Autodesk Inventor part; units mm, degrees
ref_plane "YZ Plane" through (0, 0, 0) normal (1, 0, 0) x (0, 1, 0)
ref_plane "XZ Plane" through (0, 0, 0) normal (0, 1, 0) x (-1, 0, 0)
ref_plane "XY Plane" through (0, 0, 0) normal (0, 0, 1) x (1, 0, 0)
sketch "Эскиз1" plane through (0, 0, 0) normal (1, 0, 0) x (0, 1, 0)
  circle A0 centre (0, 0) radius 60
  point P0 (0, -60)
extrude "Выдавливание1" add sketch "Эскиз1" along normal blind 4
sketch "Эскиз2" plane through (4, 0, 0) normal (1, 0, 0) x (0, 0, -1)
  point P0 (0, 0)
  point P1 (0, -60)
sketch "Эскиз3" plane through (4, 0, 0) normal (1, 0, 0) x (0, 0, -1)
  line L0 (0, -92.75) -> (0, 85.4583) construction
  circle A0 centre (0, 0) radius 60 construction
  line L1 (40.5908, -40.3227) -> (46.095, -31.9738)
  line L2 (46.095, -31.9738) -> (42.7554, -29.7722)
  line L3 (42.7554, -29.7722) -> (37.2513, -38.1211)
  line L4 (37.2513, -38.1211) -> (40.5908, -40.3227)
  line L5 (40.5908, -40.3227) -> (42.7554, -29.7722) construction
  line L6 (46.095, -31.9738) -> (37.2513, -38.1211) construction
  line L7 (41.6731, -35.0475) -> (44.4252, -30.873) construction
  line L8 (31.7471, -46.47) -> (48.2596, -21.4233) construction
  line L9 (48.2596, -21.4233) -> (51.5992, -23.6249) construction
  line L10 (51.5992, -23.6249) -> (35.0866, -48.6716) construction
  line L11 (35.0866, -48.6716) -> (31.7471, -46.47) construction
  line L12 (31.7471, -46.47) -> (51.5992, -23.6249) construction
  line L13 (48.2596, -21.4233) -> (35.0866, -48.6716) construction
  circle A1 centre (0, 0) radius 60
  line L14 (48.3995, -11.3168) -> (48.3995, -1.3168)
  line L15 (48.3995, -1.3168) -> (52.3995, -1.3168)
  line L16 (52.3995, -1.3168) -> (52.3995, -11.3168) construction
  line L17 (52.3995, -11.3168) -> (48.3995, -11.3168)
  line L18 (48.3995, -11.3168) -> (52.3995, -1.3168) construction
  line L19 (48.3995, -1.3168) -> (52.3995, -11.3168) construction
  line L20 (48.3995, -21.3168) -> (48.3995, 8.6832) construction
  line L21 (48.3995, 8.6832) -> (52.3995, 8.6832) construction
  line L22 (52.3995, 8.6832) -> (52.3995, -21.3168)
  line L23 (52.3995, -21.3168) -> (48.3995, -21.3168) construction
  line L24 (48.3995, -21.3168) -> (52.3995, 8.6832) construction
  line L25 (48.3995, 8.6832) -> (52.3995, -21.3168) construction
  line L26 (50.3995, -6.3168) -> (50.3995, 8.6832) construction
  line L27 (36.4646, 25.3316) -> (42.4094, 17.2905)
  line L28 (42.4094, 17.2905) -> (45.6259, 19.6684)
  line L29 (45.6259, 19.6684) -> (39.6811, 27.7095)
  line L30 (39.6811, 27.7095) -> (36.4646, 25.3316)
  line L31 (36.4646, 25.3316) -> (45.6259, 19.6684) construction
  line L32 (42.4094, 17.2905) -> (39.6811, 27.7095) construction
  line L33 (30.5198, 33.3727) -> (48.3542, 9.2494) construction
  line L34 (48.3542, 9.2494) -> (51.5707, 11.6273) construction
  line L35 (51.5707, 11.6273) -> (33.7363, 35.7506) construction
  line L36 (33.7363, 35.7506) -> (30.5198, 33.3727) construction
  line L37 (30.5198, 33.3727) -> (51.5707, 11.6273) construction
  line L38 (48.3542, 9.2494) -> (33.7363, 35.7506) construction
  line L39 (41.0453, 22.5) -> (32.1281, 34.5617) construction
  line L40 (10.536, 42.571) -> (20.3099, 40.4564)
  line L41 (20.3099, 40.4564) -> (19.464, 36.5468)
  line L42 (19.464, 36.5468) -> (9.6901, 38.6615)
  line L43 (9.6901, 38.6615) -> (10.536, 42.571)
  line L44 (10.536, 42.571) -> (19.464, 36.5468) construction
  line L45 (20.3099, 40.4564) -> (9.6901, 38.6615) construction
  line L46 (-0.0837, 40.7762) -> (29.2378, 34.4321) construction
  line L47 (29.2378, 34.4321) -> (30.0837, 38.3417) construction
  line L48 (30.0837, 38.3417) -> (0.7622, 44.6857) construction
  line L49 (0.7622, 44.6857) -> (-0.0837, 40.7762) construction
  line L50 (-0.0837, 40.7762) -> (30.0837, 38.3417) construction
  line L51 (29.2378, 34.4321) -> (0.7622, 44.6857) construction
  line L52 (0.3392, 42.7309) -> (15, 39.5589) construction
  line L53 (-20.2765, 33.1516) -> (-11.9215, 38.6465)
  line L54 (-11.9215, 38.6465) -> (-9.7235, 35.3046)
  line L55 (-9.7235, 35.3046) -> (-18.0785, 29.8096)
  line L56 (-18.0785, 29.8096) -> (-20.2765, 33.1516)
  line L57 (-20.2765, 33.1516) -> (-9.7235, 35.3046) construction
  line L58 (-11.9215, 38.6465) -> (-18.0785, 29.8096) construction
  line L59 (-26.4334, 24.3146) -> (-1.3686, 40.7995) construction
  line L60 (-1.3686, 40.7995) -> (-3.5666, 44.1415) construction
  line L61 (-3.5666, 44.1415) -> (-28.6314, 27.6566) construction
  line L62 (-28.6314, 27.6566) -> (-26.4334, 24.3146) construction
  line L63 (-26.4334, 24.3146) -> (-3.5666, 44.1415) construction
  line L64 (-1.3686, 40.7995) -> (-28.6314, 27.6566) construction
  line L65 (-15, 34.2281) -> (-2.4676, 42.4705) construction
  line L66 (-32.897, 9.0632) -> (-30.5956, 18.7948)
  line L67 (-30.5956, 18.7948) -> (-26.703, 17.8742)
  line L68 (-26.703, 17.8742) -> (-29.0044, 8.1427)
  line L69 (-29.0044, 8.1427) -> (-32.897, 9.0632)
  line L70 (-32.897, 9.0632) -> (-26.703, 17.8742) construction
  line L71 (-30.5956, 18.7948) -> (-29.0044, 8.1427) construction
  line L72 (-34.0478, 4.1975) -> (-29.4449, 23.6606) construction
  line L73 (-29.4449, 23.6606) -> (-25.5522, 22.74) construction
  line L74 (-25.5522, 22.74) -> (-30.1551, 3.2769) construction
  line L75 (-30.1551, 3.2769) -> (-34.0478, 4.1975) construction
  line L76 (-34.0478, 4.1975) -> (-25.5522, 22.74) construction
  line L77 (-29.4449, 23.6606) -> (-30.1551, 3.2769) construction
  line L78 (-29.8, 13.4687) -> (-27.4986, 23.2003) construction
  line L79 (-30.1437, 1.6896) -> (-20.3668, -15.7578) construction
  line L80 (-20.3668, -15.7578) -> (-23.8563, -17.7132) construction
  line L81 (-23.8563, -17.7132) -> (-33.6332, -0.2658) construction
  line L82 (-33.6332, -0.2658) -> (-30.1437, 1.6896) construction
  line L83 (-30.1437, 1.6896) -> (-23.8563, -17.7132) construction
  line L84 (-20.3668, -15.7578) -> (-33.6332, -0.2658) construction
  line L85 (-27.6995, -2.6723) -> (-22.811, -11.396)
  line L86 (-22.811, -11.396) -> (-26.3005, -13.3514)
  line L87 (-26.3005, -13.3514) -> (-31.189, -4.6277)
  line L88 (-31.189, -4.6277) -> (-27.6995, -2.6723)
  line L89 (-27.6995, -2.6723) -> (-26.3005, -13.3514) construction
  line L90 (-22.811, -11.396) -> (-31.189, -4.6277) construction
  line L91 (-27, -8.0118) -> (-31.8884, 0.7119) construction
  line L92 (-19.4768, -16.8116) -> (0.1967, -20.411) construction
  line L93 (0.1967, -20.411) -> (-0.5232, -24.3456) construction
  line L94 (-0.5232, -24.3456) -> (-20.1967, -20.7463) construction
  line L95 (-20.1967, -20.7463) -> (-19.4768, -16.8116) construction
  line L96 (-19.4768, -16.8116) -> (-0.5232, -24.3456) construction
  line L97 (0.1967, -20.411) -> (-20.1967, -20.7463) construction
  line L98 (-14.5584, -17.7114) -> (-4.7217, -19.5111)
  line L99 (-4.7217, -19.5111) -> (-5.4416, -23.4458)
  line L100 (-5.4416, -23.4458) -> (-15.2783, -21.6461)
  line L101 (-15.2783, -21.6461) -> (-14.5584, -17.7114)
  line L102 (-14.5584, -17.7114) -> (-5.4416, -23.4458) construction
  line L103 (-4.7217, -19.5111) -> (-15.2783, -21.6461) construction
  line L104 (-10, -20.5786) -> (-19.8367, -18.7789) construction
  line L105 (11.0144, -9.2398) -> (0.2107, -19.6457) construction
  line L106 (0.2107, -19.6457) -> (2.9856, -22.5267) construction
  line L107 (2.9856, -22.5267) -> (13.7893, -12.1208) construction
  line L108 (13.7893, -12.1208) -> (11.0144, -9.2398) construction
  line L109 (11.0144, -9.2398) -> (2.9856, -22.5267) construction
  line L110 (0.2107, -19.6457) -> (13.7893, -12.1208) construction
  line L111 (9.2138, -10.9742) -> (2.0113, -17.9114)
  line L112 (2.0113, -17.9114) -> (4.7862, -20.7923)
  line L113 (4.7862, -20.7923) -> (11.9887, -13.8551)
  line L114 (11.9887, -13.8551) -> (9.2138, -10.9742)
  line L115 (9.2138, -10.9742) -> (4.7862, -20.7923) construction
  line L116 (2.0113, -17.9114) -> (11.9887, -13.8551) construction
  line L117 (7, -15.8832) -> (10.6012, -12.4146) construction
  line L118 (10.3281, -8.9147) -> (8.5366, 0.9236)
  line L119 (8.5366, 0.9236) -> (12.4719, 1.6401)
  line L120 (12.4719, 1.6401) -> (14.2634, -8.1981)
  line L121 (14.2634, -8.1981) -> (10.3281, -8.9147)
  line L122 (10.3281, -8.9147) -> (12.4719, 1.6401) construction
  line L123 (8.5366, 0.9236) -> (14.2634, -8.1981) construction
  line L124 (10.3281, -8.9147) -> (8.5366, 0.9236)
  line L125 (8.5366, 0.9236) -> (12.4719, 1.6401)
  line L126 (12.4719, 1.6401) -> (14.2634, -8.1981)
  line L127 (14.2634, -8.1981) -> (10.3281, -8.9147)
  line L128 (10.3281, -8.9147) -> (12.4719, 1.6401) construction
  line L129 (8.5366, 0.9236) -> (14.2634, -8.1981) construction
  line L130 (11.4, -3.6373) -> (10.5043, 1.2819) construction
  line L131 (-0.9405, 1.4271) -> (9.0554, 1.7143)
  line L132 (9.0554, 1.7143) -> (8.9405, 5.7126)
  line L133 (8.9405, 5.7126) -> (-1.0554, 5.4255)
  line L134 (-1.0554, 5.4255) -> (-0.9405, 1.4271)
  line L135 (-0.9405, 1.4271) -> (8.9405, 5.7126) construction
  line L136 (9.0554, 1.7143) -> (-1.0554, 5.4255) construction
  line L137 (-0.9405, 1.4271) -> (9.0554, 1.7143)
  line L138 (9.0554, 1.7143) -> (8.9405, 5.7126)
  line L139 (8.9405, 5.7126) -> (-1.0554, 5.4255)
  line L140 (-1.0554, 5.4255) -> (-0.9405, 1.4271)
  line L141 (-0.9405, 1.4271) -> (8.9405, 5.7126) construction
  line L142 (9.0554, 1.7143) -> (-1.0554, 5.4255) construction
  line L143 (4, 3.5699) -> (-0.9979, 3.4263) construction
  line L144 (3.8726, -59.8749) -> (32.3753, -50.5157) construction
  line L145 (32.3753, -50.5157) -> (31.1274, -46.7154) construction
  line L146 (31.1274, -46.7154) -> (2.6247, -56.0745) construction
  line L147 (2.6247, -56.0745) -> (3.8726, -59.8749) construction
  line L148 (3.8726, -59.8749) -> (31.1274, -46.7154) construction
  line L149 (32.3753, -50.5157) -> (2.6247, -56.0745) construction
  line L150 (13.3735, -56.7552) -> (22.8744, -53.6355)
  line L151 (22.8744, -53.6355) -> (21.6265, -49.8351)
  line L152 (21.6265, -49.8351) -> (12.1256, -52.9548)
  line L153 (12.1256, -52.9548) -> (13.3735, -56.7552)
  line L154 (13.3735, -56.7552) -> (21.6265, -49.8351) construction
  line L155 (22.8744, -53.6355) -> (12.1256, -52.9548) construction
  line L156 (17.5, -53.2951) -> (31.7514, -48.6155) construction
  point P0 (0, -60)
  point P1 (50.3995, -6.3168)
  point P2 (41.0453, 22.5)
  point P3 (15, 39.5589)
  point P4 (15, 39.5589)
  point P5 (-15, 34.2281)
  point P6 (-15, 34.2281)
  point P7 (-15, 34.2281)
  point P8 (-29.8, 13.4687)
  point P9 (-29.8, 13.4687)
  point P10 (-27, -8.0118)
  point P11 (-27, -8.0118)
  point P12 (-10, -20.5786)
  point P13 (7, -15.8832)
  point P14 (7, -15.8832)
  point P15 (11.4, -3.6373)
  point P16 (4, 3.5699)
  point P17 (4, 3.5699)
  point P18 (17.5, -53.2951)
  dimension "d83" = 0
  dimension "d84" = 1
  dimension "d93" = 10
  dimension "d94" = 4
  dimension "d95" = 30
  dimension "d96" = 10
  dimension "d98" = 4
  dimension "d99" = 30
  dimension "d100" = 10
  dimension "d101" = 30
  dimension "d102" = 4
  dimension "d103" = 22.5
  dimension "d104" = 10
  dimension "d105" = 30
  dimension "d106" = 4
  dimension "d107" = 15
  dimension "d108" = 30
  dimension "d109" = 4
  dimension "d110" = 10
  dimension "d111" = 15
  dimension "d112" = 10
  dimension "d113" = 20
  dimension "d114" = 4
  dimension "d115" = 29.8
  dimension "d116" = 20
  dimension "d117" = 10
  dimension "d118" = 4
  dimension "d119" = 27
  dimension "d120" = 10
  dimension "d121" = 20
  dimension "d122" = 4
  dimension "d123" = 10
  dimension "d124" = 10
  dimension "d125" = 15
  dimension "d127" = 4
  dimension "d128" = 7
  dimension "d132" = 10
  dimension "d134" = 4
  dimension "d135" = 10
  dimension "d136" = 11.4
  dimension "d137" = 10
  dimension "d138" = 10
  dimension "d139" = 4
  dimension "d140" = 4
  dimension "d141" = 4
  dimension "d142" = 30
  dimension "d143" = 10
  dimension "d144" = 17.5
extrude "Выдавливание2" cut sketch "Эскиз3" against normal through all contours L4 L3 L2 L1 | L14 L15 L22 L17 | L30 L29 L28 L27 | L40 L41 L42 L43 | L53 L54 L55 L56 | L66 L67 L68 L69 | L85 L86 L87 L88 | L98 L99 L100 L101 | L114 L113 L112 L111 | L118 L119 L120 L121 | L153 L152 L151 L150
properties part number "Стенка барабана"
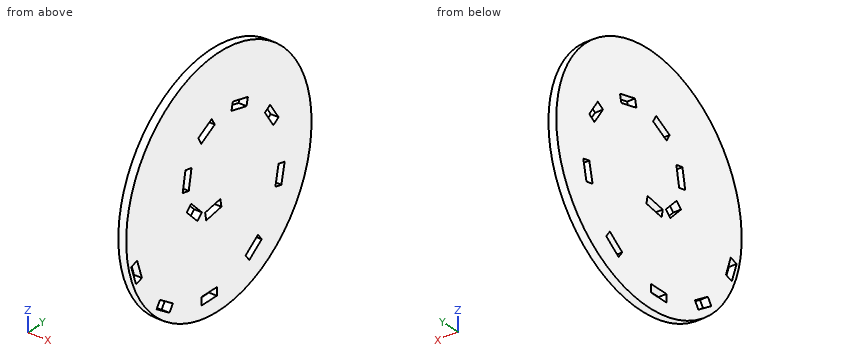
Check sheet for the modelled part. Datum: model origin and axes. Units: mm. Give positions to 0.01 mm unless a question says otherwise; leave off trailing zeros. Order: outer loops, then holes, each group sorted by start corner. A loop starts at its lowest first (then second) coordinate and runs counter-clockwise, first axis right, second up. Notation, with made-up numbers: (-11.5, 74.5) -> (21.5, 74.5) arc R24 cw to (21.5, 105.5) -> close; hole circle Ø10 at (-28.75, -19.5). An arc over 180 degrees is marked (long way). Use CSV: the item, a comma, the result in double quotes. Start each with the question number.
1) Sectioned sample at C-C, the plane z = -33. Record the boundary of the cut face in (x, y).
2) Sectioned sample at A-A, the plane x = 1. Give the number of separate pieces and of enclosed holes in the cut face, plus the area to 3 significant figures.
3) Sectioned sample at B-B, the plane y = 45. Record the boundary of the cut face in (x, z), plus the area to 3 significant figures.
4) Go/stop test with flat-tipped pins: P1, Ø1.2, axis at x = 2.5, z = -51.5, coming from the -Y side; P2, Ø1.5, axis at x = 2.5, y = -11.5, coming from the -Z side. Record where each tip stops, or that it passes through.
5) Material ranges on line 1 (Z direction, x = 1.95, y = -4); line 2 (Z direction, x = 3.25, y = -20); line 3 (Y direction, x = 2.5, z = 9), recorded low to high. Write a range as from..to.
Recorded:
1,outline,"(0, -50.11) -> (4, -50.11) -> (4, 50.11) -> (0, 50.11) -> close"
2,separate pieces,"1"
2,enclosed holes,"11"
2,area,"10,900 mm2"
3,outline,"(0, -39.69) -> (4, -39.69) -> (4, 39.69) -> (0, 39.69) -> close"
3,area,"317 mm2"
4,P1,"y = -31.77"
4,P2,"z = -59.03"
5,line 1,"-59.87..-52.4, -48.4..-13.5, -9.43..26.96, 30.07..59.87"
5,line 2,"-56.57..-5.61, -4.02..4.81, 14.98..56.57"
5,line 3,"-59.32..-22.79, -18.73..59.32"
